```python
from build123d import *

# Parameters (mm, degrees)
SKETCH1_W           = 16
SKETCH1_H           = 30
SKETCH1_R           = 4.2
BOSS_EXTRUDE1_DEPTH = 5
SKETCH2_W           = 11
SKETCH2_H           = 26
SKETCH2_R           = 1.75
BOSS_EXTRUDE2_DEPTH = 9
SKETCH3_W           = 16
SKETCH3_H           = 13
BOSS_EXTRUDE3_DEPTH = 8
CUT_EXTRUDE1_START  = 1
CUT_EXTRUDE1_DEPTH  = 4
CUT_EXTRUDE2_DEPTH  = 7
FILLET1_START       = -10
FILLET1_DEPTH       = 10
FILLET1_START_2     = 5
FILLET1_2_DEPTH     = 9
FILLET1_START_3     = -6
FILLET1_3_DEPTH     = 11


with BuildPart() as part:
    # Sketch1 → Boss-Extrude1 (new body)
    with BuildSketch(Plane(origin=(0, 0, 0), x_dir=(0, 0, -1), z_dir=(1, 0, 0))):
        with Locations((8, -15)):
            Rectangle(SKETCH1_W, SKETCH1_H)
        with Locations((8, -20)):
            Circle(SKETCH1_R, mode=Mode.SUBTRACT)
    extrude(amount=BOSS_EXTRUDE1_DEPTH)

    # Sketch2 → Boss-Extrude2 (add)
    with BuildSketch(Plane.XY):
        with Locations((-0.5, 13)):
            Rectangle(SKETCH2_W, SKETCH2_H)
        with Locations((-3.25, 22.25)):
            Circle(SKETCH2_R, mode=Mode.SUBTRACT)
        with Locations((-3.25, 3.25)):
            Circle(SKETCH2_R, mode=Mode.SUBTRACT)
    extrude(amount=-BOSS_EXTRUDE2_DEPTH)

    # Sketch3 → Boss-Extrude3 (add)
    with BuildSketch(Plane(origin=(5, 0, 0), x_dir=(0, 0, -1), z_dir=(1, 0, 0))):
        with Locations((8, -6.5)):
            Rectangle(SKETCH3_W, SKETCH3_H)
    extrude(amount=BOSS_EXTRUDE3_DEPTH)

    # Sketch5 → Cut-Extrude1 (cut)
    with BuildSketch(Plane(origin=(5, 0, 0), x_dir=(0, 0, -1), z_dir=(1, 0, 0)).offset(CUT_EXTRUDE1_START)):
        with BuildLine():
            ThreePointArc((3, -6.5), (3.288161187, -8.172894198), (4.119429999, -9.652963125))
            Line((4.119429999, -9.652963125), (11.880570001, -3.347036875))
            ThreePointArc((11.880570001, -3.347036875), (6.327105802, -1.788161187), (3, -6.5))
        make_face()
        with BuildLine():
            Line((11.880570001, -3.347036875), (4.119429999, -9.652963125))
            ThreePointArc((4.119429999, -9.652963125), (9.672894198, -11.211838813), (13, -6.5))
            ThreePointArc((13, -6.5), (12.711838813, -4.827105802), (11.880570001, -3.347036875))
        make_face()
        with BuildLine():
            ThreePointArc((3, -6.5), (6.327105802, -1.788161187), (11.880570001, -3.347036875))
            Line((11.880570001, -3.347036875), (13, -2.4375))
            Line((13, -2.4375), (13, 0))
            Line((13, 0), (9, 0))
            Line((9, 0), (3, 0))
            Line((3, 0), (3, -6.5))
        make_face()
        with BuildLine():
            Line((13, -2.4375), (11.880570001, -3.347036875))
            ThreePointArc((11.880570001, -3.347036875), (12.711838813, -4.827105802), (13, -6.5))
            Line((13, -6.5), (13, -2.4375))
        make_face()
    extrude(amount=CUT_EXTRUDE1_DEPTH, mode=Mode.SUBTRACT)

    # Sketch6 → Cut-Extrude2 (cut)
    with BuildSketch(Plane(origin=(13, 0, 0), x_dir=(0, 0, -1), z_dir=(1, 0, 0))):
        with BuildLine():
            Line((10.3, 0), (5.7, 0))
            Line((5.7, 0), (5.7, -6.5))
            ThreePointArc((5.7, -6.5), (8, -8.8), (10.3, -6.5))
            Line((10.3, -6.5), (10.3, 0))
        make_face()
    extrude(amount=-CUT_EXTRUDE2_DEPTH, mode=Mode.SUBTRACT)

    # Fillet1: read off the stored shape, not the designer's step
    # Fillet1 outline → Fillet1 (cut)
    with BuildSketch(Plane.XY.offset(FILLET1_START)):
        with BuildLine():
            Line((-6, 26), (-6, 23))
            ThreePointArc((-6, 23), (-5.121320344, 25.121320344), (-3, 26))
            Line((-3, 26), (-6, 26))
        make_face()
        with BuildLine():
            ThreePointArc((-3, 0), (-5.121320344, 0.878679656), (-6, 3))
            Line((-6, 3), (-6, 0))
            Line((-6, 0), (-3, 0))
        make_face()
        with BuildLine():
            Line((5, 26), (2, 26))
            ThreePointArc((2, 26), (4.121320344, 25.121320344), (5, 23))
            Line((5, 23), (5, 26))
        make_face()
    extrude(amount=FILLET1_DEPTH, mode=Mode.SUBTRACT)

    # Fillet1 2 outline → Fillet1 2 (cut)
    with BuildSketch(Plane.YZ.offset(FILLET1_START_2)):
        with BuildLine():
            Line((0, 0), (-3, 0))
            ThreePointArc((-3, 0), (-0.878679656, -0.878679656), (0, -3))
            Line((0, -3), (0, 0))
        make_face()
        with BuildLine():
            ThreePointArc((-13, -3), (-12.121320344, -0.878679656), (-10, 0))
            Line((-10, 0), (-13, 0))
            Line((-13, 0), (-13, -3))
        make_face()
        with BuildLine():
            Line((0, -16), (0, -13))
            ThreePointArc((0, -13), (-0.878679656, -15.121320344), (-3, -16))
            Line((-3, -16), (0, -16))
        make_face()
        with BuildLine():
            ThreePointArc((-10, -16), (-12.121320344, -15.121320344), (-13, -13))
            Line((-13, -13), (-13, -16))
            Line((-13, -16), (-10, -16))
        make_face()
    extrude(amount=FILLET1_2_DEPTH, mode=Mode.SUBTRACT)

    # Fillet1 3 outline → Fillet1 3 (cut)
    with BuildSketch(Plane.YZ.offset(FILLET1_START_3)):
        with BuildLine():
            Line((0, -16), (0, -13))
            ThreePointArc((0, -13), (-0.878679656, -15.121320344), (-3, -16))
            Line((-3, -16), (0, -16))
        make_face()
        with BuildLine():
            ThreePointArc((-30, -3), (-29.121320344, -0.878679656), (-27, 0))
            Line((-27, 0), (-30, 0))
            Line((-30, 0), (-30, -3))
        make_face()
        with BuildLine():
            Line((-30, -16), (-27, -16))
            ThreePointArc((-27, -16), (-29.121320344, -15.121320344), (-30, -13))
            Line((-30, -13), (-30, -16))
        make_face()
    extrude(amount=FILLET1_3_DEPTH, mode=Mode.SUBTRACT)


solid = part.part
```
Could you check a few things on this model? Use its own coordinates, in mm. A direction names the side the tool comes from. Give positions to 0.01 mm unless a question says otherwise; leave off trailing zeros. Write each loop counter-clockwise with the first axis right and the second up, starting at its lowest first coordinate (ties: lowest second). Pieces come first, ordered by that corner, then holes. Notation, with made-up numbers: (-37.75, 69.5) - (-30.75, 69.5) arc R29 cw to (-30.75, 105.5) - close; hole circle Ø7 at (20.25, -33.75). An arc over 180 degrees is marked (long way). One line per item, written item: value. Start each with the question number.
Item 1: If we mould it in two halves opening along Z, with no side actions, what happens to faces 1 (the face through (-2, 0, -4)), 2 (the face through (2.46, -29.1, -15.14)), 3 (the face through (10, -8, -6))? For each: +Z half, -Z half, draft (parallel to the pull), parting line (faces both ways), or undercut.
Item 2: Imagine slicing it at A-A, the plane z = -8. List the corners of the cut face in (x, y) for me, and give its area (3 significant figures).
Item 3: Please list where these lines run through material, in increasing order: line 1 (Y direction, x = -3.25, z = -3.5); line 2 (Z direction, x = -3.5, y = 15); line 3 (X direction, y = -6, z = -2.25). Write a range as from..to.
Item 4: Which directions (+Z, -Z, +X, -X, +Y, -Y) give clear straight access to the entire face, cutting with the end or side of a thin tool? Please do faces 4 (the face through (9, -13, -8)), 5 (the face through (0, -15, -8)), 6 (the face through (-1, 13, -9)), 7 (the face through (6, -6, -8)).
Item 5: Imagine slicing it at B-B, the plane y = 22.25. List the corners of the cut face in (x, z) for me, and give its area (3 significant figures).
Item 6: Imagine slicing it at D-D, the plane z = -11.5. List the corners of the cut face in (x, y) for me, and give its area (3 significant figures).
Item 7: I'm going to push flat-ended pins straight in: pin 1 (1.5 mm diameter, centred on x = -1, z = -4, fed in from -Y); pin 2 (2 mm diameter, centred on x = 8, z = -10.5, fed in from -Y); pin 3 (2.5 mm diameter, centred on y = 13.5, z = -3, fed in from +X). Where does each tip first touch, or does it pass through?
Item 8: Imagine slicing it at C-C, the plane x = 10.75. List the corners of the cut face in (y, z) for me, and give its area (3 significant figures).
Geometry says:
1. face 1: draft
1. face 2: -Z half
1. face 3: undercut
2. outline: (-6, 3) arc R3 ccw to (-3, 0) - (0, 0) - (0, -15.8) - (5, -15.8) - (5, -13) - (13, -13) - (13, -8.8) - (10, -8.8) - (10, -11.5) - (6, -11.5) - (6, 0) - (5, 0) - (5, 23) arc R3 ccw to (2, 26) - (-3, 26) arc R3 ccw to (-6, 23) - close; (0, -30) - (5, -30) - (5, -24.2) - (0, -24.2) - close; hole circle Ø3.5 at (-3.25, 3.25); hole circle Ø3.5 at (-3.25, 22.25)
2. area: 401 mm^2
3. line 1: 0.01..1.5, 5..20.5, 24..25.99
3. line 2: -9..0
3. line 3: 0..13
4. face 4: +Z, -Z, +X, -Y
4. face 5: +Z, -Z, -X, -Y
4. face 6: -Z, +X, -X, +Y
4. face 7: +Y
5. outline: (-6, -9) - (-5, -9) - (-5, 0) - (-6, 0) - close; (-1.5, -9) - (5, -9) - (5, 0) - (-1.5, 0) - close
5. area: 67.5 mm^2
6. outline: (0, -30) - (5, -30) - (5, -22.32) - (0, -22.32) - close; (0, -17.68) - (5, -17.68) - (5, -13) - (13, -13) - (13, 0) - (10, 0) - (10, -10.07) - (6, -10.07) - (6, 0) - (0, 0) - close
6. area: 191 mm^2
7. pin 1: y = 0
7. pin 2: y = -13
7. pin 3: x = 5
8. outline: (-13, -13) arc R3 ccw to (-10, -16) - (-3, -16) arc R3 ccw to (0, -13) - (0, -10.3) - (-6.5, -10.3) arc R2.3 cw to (-6.5, -5.7) - (0, -5.7) - (0, -3) arc R3 ccw to (-3, 0) - (-10, 0) arc R3 ccw to (-13, -3) - close
8. area: 162 mm^2
